from build123d import *

# Parameters (mm, degrees)
SKETCH1_R           = 28.575
SKETCH1_R_2         = 3.96875
BOSS_EXTRUDE1_DEPTH = 3.175
SKETCH2_R           = 3.96875
CUT_EXTRUDE1_DEPTH  = 41.535686438
CIRPATTERN1_COUNT   = 4


with BuildPart() as part:
    # Sketch1 → Boss-Extrude1 (new body)
    with BuildSketch(Plane(origin=(0, 0, 0), x_dir=(0, 0, -1), z_dir=(1, 0, 0))):
        Circle(SKETCH1_R)
        Circle(SKETCH1_R_2, mode=Mode.SUBTRACT)
    extrude(amount=BOSS_EXTRUDE1_DEPTH)

    # Sketch2 → Cut-Extrude1 (cut, through all)
    with BuildSketch(Plane(origin=(0, 0, 0), x_dir=(0, 0, -1), z_dir=(1, 0, 0))):
        with Locations((0, 19.05)):
            Circle(SKETCH2_R)
    cut_extrude1 = extrude(amount=CUT_EXTRUDE1_DEPTH, mode=Mode.SUBTRACT)

    # CirPattern1: Cut-Extrude1 ×4 about axis
    cirpattern1_axis = Axis((0, 0, 0), (1, 0, 0))
    for i in range(1, CIRPATTERN1_COUNT):
        add(cut_extrude1.rotate(cirpattern1_axis, i * 360 / CIRPATTERN1_COUNT), mode=Mode.SUBTRACT)


solid = part.part
Geometry check sheet. Reference: the model listing, model coordinates, mm. Give positions to 0.01 mm unless a question says otherwise; leave off trailing zeros. Order: outer loops, then holes, each group sorted by start corner. A loop starts at its lowest first (then second) coordinate and runs counter-clockwise, first axis right, second up. Notation, with made-up numbers: M -31.5,19 L -22.5,19 A17 cw -22.5,32 Z; hole C 26.25,71.5 d4. An arc over 180 degrees is marked long. Use a Markdown table: item, result.
Item 1: Depth check by flat-ended pin: P1, Ø1, axis at x = 2, z = -17, coming from the -Y side; P2, Ø1, axis at x = 1.5, z = -3.5, coming from the -Y side. Enter the tip coordinate at first touch or a pass-through.
Answers follow:
| item | result |
|---|---|
| P1 | stops at y = -23.33 |
| P2 | stops at y = -28.42 |
Item 2: Section check D-D (x = 1.35). State how many separate pieces and enclosed holes the cut face has, and give its area (3 significant figures).
Answers follow:
| item | result |
|---|---|
| separate pieces | 1 |
| enclosed holes | 5 |
| area | 2,320 mm2 |
Item 3: Draft check along Y on faces 1 (the cylindrical face through (1.565, -3.874, 0.86)), 2 (the cylindrical face through (1.565, -0.517, 22.985)), 3 (the cylindrical face through (1.565, 1.256, 28.547)), 4 (the flat face through (0, -6, 0)). Enter one of: +Y half, -Y half, draft (parallel to the pull), parting line (faces both ways), or undercut.
Answers follow:
| item | result |
|---|---|
| face 1 | undercut |
| face 2 | undercut |
| face 3 | parting line |
| face 4 | draft |
Item 4: Section check C-C (z = -16.5). Record the cut outline in (x, y) (3 decimals).
Answers follow:
| item | result |
|---|---|
| outline | M 0,-23.33 L 3.175,-23.33 L 3.175,-3.041 L 0,-3.041 Z; M 0,3.041 L 3.175,3.041 L 3.175,23.33 L 0,23.33 Z |
Item 5: Section check A-A (z = 0). Record the cut outline in (x, y) (3 decimals).
Answers follow:
| item | result |
|---|---|
| outline | M 0,-28.575 L 3.175,-28.575 L 3.175,-23.019 L 0,-23.019 Z; M 0,-15.081 L 3.175,-15.081 L 3.175,-3.969 L 0,-3.969 Z; M 0,3.969 L 3.175,3.969 L 3.175,15.081 L 0,15.081 Z; M 0,23.019 L 3.175,23.019 L 3.175,28.575 L 0,28.575 Z |
Item 6: Material ranges on line 1 along Y through (x, z) = (1.3, 0) (3 decimals); line 2 along Z through (x, y) = (2.8, 2); line 3 along Y through (x, z) = (1.5, -15.5), recorded low to high.
Answers follow:
| item | result |
|---|---|
| line 1 | y = -28.575 to -23.019, -15.081 to -3.969, 3.969 to 15.081, 23.019 to 28.575 |
| line 2 | z = -28.5 to -22.48, -15.62 to -3.43, 3.43 to 15.62, 22.48 to 28.5 |
| line 3 | y = -24.01 to -1.77, 1.77 to 24.01 |
Item 7: Section check B-B (y = -2.5). Record the cut outline in (x, z) (3 decimals).
Answers follow:
| item | result |
|---|---|
| outline | M 0,-28.465 L 3.175,-28.465 L 3.175,-22.132 L 0,-22.132 Z; M 0,-15.968 L 3.175,-15.968 L 3.175,-3.082 L 0,-3.082 Z; M 0,3.082 L 3.175,3.082 L 3.175,15.968 L 0,15.968 Z; M 0,22.132 L 3.175,22.132 L 3.175,28.465 L 0,28.465 Z |
